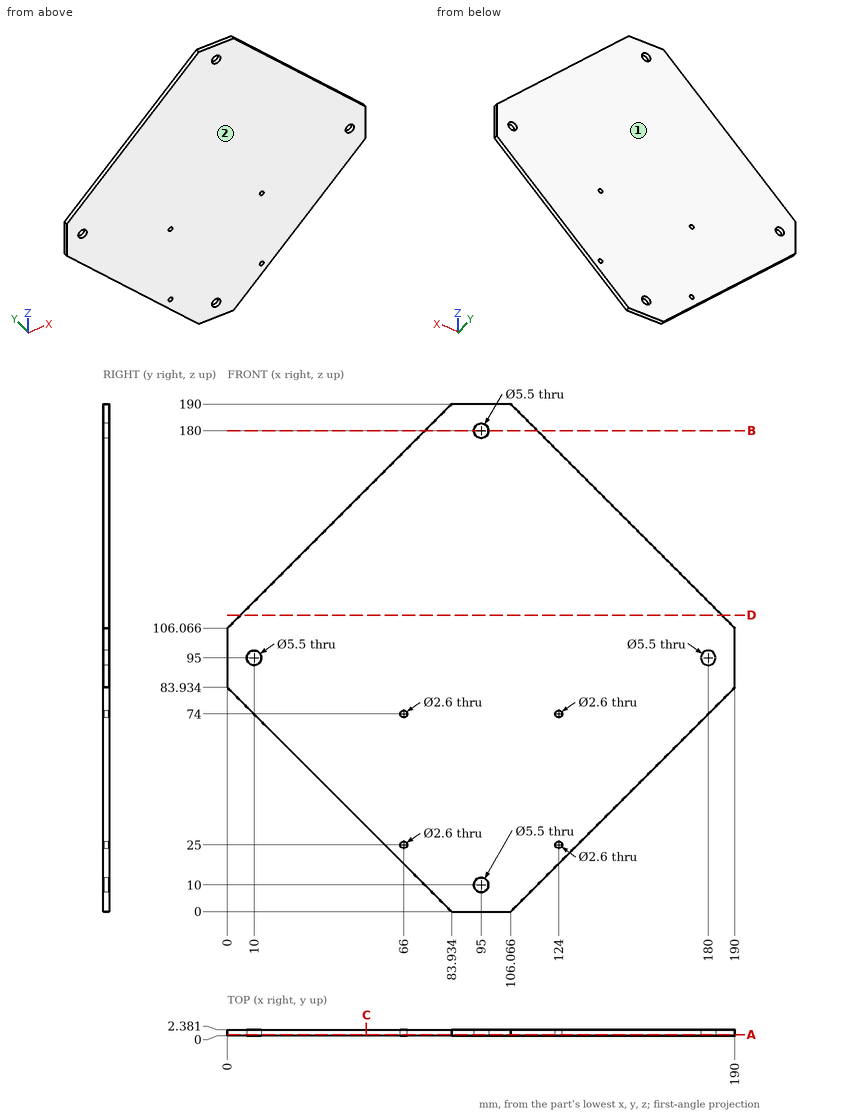
Check sheet for the drawn part. Datum: minimum x, y, z corner. Units: mm. Coordinates: 2 decimals unless noted, no trailing zeros. Loops run counter-clockwise (first coordinate to the right, second up) from the corner with the lowest first, then second, coordinate; pieces in that order, holes last. Notation, with made-up numbers: (-6.75, 74) -> (44.25, 74) arc R23 ccw to (44.25, 89) -> close; hole circle Ø7 at (-4, -37.5). An arc over 180 degrees is marked (long way). Answer in a Markdown table with one row per item.
1) Section check D-D (z = 111). Record the cut outline in (x, y).
The answers:
| item | result |
|---|---|
| outline | (4.93, 0) -> (185.07, 0) -> (185.07, 2.38) -> (4.93, 2.38) -> close |
2) Section check C-C (x = 52). Record the cut outline in (y, z).
The answers:
| item | result |
|---|---|
| outline | (0, 31.93) -> (2.38, 31.93) -> (2.38, 158.07) -> (0, 158.07) -> close |
3) Draft check along Y on the marked faces 1 and 2. Enter one of: released by +Y, released by -Y, zero draft, split by the parting line, or undercut.
The answers:
| item | result |
|---|---|
| face 1 | released by +Y |
| face 2 | released by -Y |
4) Section check A-A (y = 0.55). Give the number of separate pieces and of enclosed holes in the cut face, and give its area (3 significant figures).
The answers:
| item | result |
|---|---|
| separate pieces | 1 |
| enclosed holes | 8 |
| area | 21,900 mm2 |
5) Section check B-B (z = 180). Record the cut outline in (x, y).
The answers:
| item | result |
|---|---|
| outline | (73.93, 0) -> (92.25, 0) -> (92.25, 2.38) -> (73.93, 2.38) -> close; (97.75, 0) -> (116.07, 0) -> (116.07, 2.38) -> (97.75, 2.38) -> close |
6) Depth check by flat-ended pin: P1, Ø5, axis at x = 95, z = 180, coming from the -Y side; P2, Ø1, axis at x = 115.5, y = 2, coming from the -Z side (1 decimal); P3, Ø7, axis at x = 95, z = 10, coming from the -Y side; P4, Ø1, axis at y = 1, z = 168.5, coming from the -X side (1 decimal). Enter the tip coordinate at first touch or a pass-through.
The answers:
| item | result |
|---|---|
| P1 | passes through |
| P2 | stops at z = 8.9 |
| P3 | stops at y = 0 |
| P4 | stops at x = 61.9 |
7) Scan lines: line 1 along X through (y, z) = (1.2, 25) (1 decimal); line 2 along X through (y, z) = (0.8, 74) (1 decimal); line 3 along X through (y, z) = (1.45, 12.5) (1 decimal). Record each from-to range of solid material in increasing order. Write a range as from..to.
The answers:
| item | result |
|---|---|
| line 1 | x = 58.9..64.7, 67.3..122.7, 125.3..131.1 |
| line 2 | x = 9.9..64.7, 67.3..122.7, 125.3..180.1 |
| line 3 | x = 71.4..93.9, 96.1..118.6 |
